```python
from build123d import *

# Parameters (mm, degrees)
ESBO_O1_R                      = 1.5
RESSALTO_EXTRUS_O1_DEPTH       = 6
ESBO_O6_W                      = 14
ESBO_O6_H                      = 22
RESSALTO_EXTRUS_O3_DEPTH       = 12
ESBO_O7_R                      = 5
CORTE_EXTRUS_O4_DEPTH          = 30.538450843
FILETE3_R                      = 5
RESSALTO_EXTRUS_O13_DEPTH      = 8
RESSALTO_EXTRUS_O13_DEPTH_BACK = 5
ESBO_O15_R                     = 2
ESBO_O17_R                     = 1
CORTE_EXTRUS_O6_DEPTH          = 8
ESBO_O21_W                     = 22.669500521
ESBO_O21_H                     = 31.157259519
CORTE_EXTRUS_O8_DEPTH          = 6
ESBO_O22_W                     = 5
ESBO_O22_H                     = 5
ESBO_O22_R                     = 1.5
RESSALTO_EXTRUS_O15_DEPTH      = 3
ESBO_O23_R                     = 2.5
RESSALTO_EXTRUS_O16_DEPTH      = 5
ESBO_O24_R                     = 0.75
CORTE_EXTRUS_O9_DEPTH          = 5
CHANFRO5_SIZE                  = 1
ESBO_O25_R                     = 1.5
CORTE_EXTRUS_O11_DEPTH         = 14


with BuildPart() as part:
    # Esboço1 → Ressalto-extrusão1 (new body)
    with BuildSketch(Plane.XY):
        Polygon((-11.637137788, -1.832768542), (5.362862212, -1.832768542), (5.362862212, 7.667231458), (10.362862212, 7.667231458), (10.362862212, 16.667231458), (5.362862212, 16.667231458), (5.362862212, 20.167231458), (-10.637137788, 20.167231458), (-10.637137788, 16.667231458), (-15.637137788, 16.667231458), (-15.637137788, 7.667231458), (-11.637137788, 7.667231458), align=None)
        with Locations((6.362862212, 11.867231458)):
            Circle(ESBO_O1_R, mode=Mode.SUBTRACT)
        with Locations((-11.637137788, 11.867231458)):
            Circle(ESBO_O1_R, mode=Mode.SUBTRACT)
    extrude(amount=RESSALTO_EXTRUS_O1_DEPTH)

    # Esboço6 → Ressalto-extrusão3 (add)
    with BuildSketch(Plane(origin=(0, 0, 0), x_dir=(-1, 0, 0), z_dir=(0, 0, -1))):
        with Locations((2.637137788, 9.167231458)):
            Rectangle(ESBO_O6_W, ESBO_O6_H)
    extrude(amount=RESSALTO_EXTRUS_O3_DEPTH)

    # Esboço7 → Corte-extrusão4 (cut, through all)
    with BuildSketch(Plane.XZ.offset(1.832768542)):
        with Locations(Location((-2.637137788, -5, 0), (0, 0, 270))):
            Circle(ESBO_O7_R)
    extrude(amount=-CORTE_EXTRUS_O4_DEPTH, mode=Mode.SUBTRACT)

    # Filete3
    filete3_edges = [part.edges().sort_by_distance(p)[0] for p in [
        (4.362862212, 9.167231458, -12),
        (-9.637137788, 9.167231458, -12),
    ]]
    fillet(filete3_edges, radius=FILETE3_R)

    # Esboço15 → Ressalto-extrusão13 (add, two sides: drawn at the far end of the back side and taken through both)
    with BuildSketch(Plane(origin=(0, 20.167231458, 0), x_dir=(1, 0, 0), z_dir=(0, 1, 0)).offset(-RESSALTO_EXTRUS_O13_DEPTH_BACK)):
        with Locations(Location((-8.650480796, 5, 0), (0, 0, 270))):
            Circle(ESBO_O15_R)
        with Locations(Location((3.376205221, 5, 0), (0, 0, 270))):
            Circle(ESBO_O15_R)
    extrude(amount=RESSALTO_EXTRUS_O13_DEPTH + RESSALTO_EXTRUS_O13_DEPTH_BACK)

    # Esboço17 → Corte-extrusão6 (cut)
    with BuildSketch(Plane(origin=(0, 28.167231458, 0), x_dir=(1, 0, 0), z_dir=(0, 1, 0))):
        with Locations(Location((-8.650480796, 5, 0), (0, 0, 270))):
            Circle(ESBO_O17_R)
        with Locations(Location((3.376205221, 5, 0), (0, 0, 270))):
            Circle(ESBO_O17_R)
    extrude(amount=-CORTE_EXTRUS_O6_DEPTH, mode=Mode.SUBTRACT)

    # Esboço21 → Corte-extrusão8 (cut)
    with BuildSketch(Plane(origin=(0, 0, -7.115225733), x_dir=(1, 0, 0), z_dir=(0, 0, -1))):
        with Locations((-2.778124877, -9.864448806)):
            Rectangle(ESBO_O21_W, ESBO_O21_H)
    extrude(amount=CORTE_EXTRUS_O8_DEPTH, mode=Mode.SUBTRACT)

    # Esboço22 → Ressalto-extrusão15 (add)
    # profile 1 of 2: a face of its own
    with BuildSketch(Plane(origin=(0, 0, -7.115225733), x_dir=(1, 0, 0), z_dir=(0, 0, -1))):
        with Locations((-12.135809914, -15.625880271)):
            Rectangle(ESBO_O22_W, ESBO_O22_H)
        with Locations(Location((-12.135809914, -15.625880271, 0), (0, 0, 180))):
            Circle(ESBO_O22_R, mode=Mode.SUBTRACT)
    # profile 2 of 2: a face of its own
    with BuildSketch(Plane(origin=(0, 0, -7.115225733), x_dir=(1, 0, 0), z_dir=(0, 0, -1))):
        with Locations((6.862862212, -15.625880271)):
            Rectangle(ESBO_O22_W, ESBO_O22_H)
        with Locations(Location((6.862862212, -15.625880271, 0), (0, 0, 180))):
            Circle(ESBO_O22_R, mode=Mode.SUBTRACT)
    extrude(amount=-RESSALTO_EXTRUS_O15_DEPTH)

    # Esboço23 → Ressalto-extrusão16 (add)
    with BuildSketch(Plane.XZ.offset(1.832768542)):
        with Locations(Location((-9.213137788, 2.7, 0), (0, 0, 165.836166317))):
            Circle(ESBO_O23_R)
    extrude(amount=RESSALTO_EXTRUS_O16_DEPTH)

    # Esboço24 → Corte-extrusão9 (cut)
    with BuildSketch(Plane.XZ.offset(6.832768542)):
        with Locations(Location((-9.213137788, 2.7, 0), (0, 0, 270))):
            Circle(ESBO_O24_R)
    extrude(amount=-CORTE_EXTRUS_O9_DEPTH, mode=Mode.SUBTRACT)

    # Chanfro5
    # the kernel refuses this chamfer: 1 mm, written as the material it takes off along each edge
    with BuildSketch(Plane(origin=(6.362862212, 11.867231458, 0), x_dir=(1, 0, 0), z_dir=(0, -1, 0))) as chanfro5_piece_1_section:
        Polygon((1.5 + CHANFRO5_SIZE, 0), (1.5, CHANFRO5_SIZE), (1.5, 0), align=None)
    chanfro5_piece_1 = revolve(axis=Axis((6.362862212, 11.867231458, 0), (0, 0, 1)), mode=Mode.PRIVATE)
    chanfro5_piece_1 = split(chanfro5_piece_1, bisect_by=Plane(origin=(4.362862212, 13.893105183, 0.134898453), z_dir=(1, 0, 0)), keep=Keep.TOP, mode=Mode.PRIVATE)
    add(chanfro5_piece_1, mode=Mode.SUBTRACT)
    with BuildSketch(Plane(origin=(-11.637137788, 11.867231458, 0), x_dir=(1, 0, 0), z_dir=(0, -1, 0))) as chanfro5_piece_2_section:
        Polygon((1.5 + CHANFRO5_SIZE, 0), (1.5, CHANFRO5_SIZE), (1.5, 0), align=None)
    chanfro5_piece_2 = revolve(axis=Axis((-11.637137788, 11.867231458, 0), (0, 0, 1)), mode=Mode.PRIVATE)
    chanfro5_piece_2 = split(chanfro5_piece_2, bisect_by=Plane(origin=(-9.637137788, 11.867231458, 0.487087965), z_dir=(-1, 0, 0)), keep=Keep.TOP, mode=Mode.PRIVATE)
    add(chanfro5_piece_2, mode=Mode.SUBTRACT)

    # Esboço25 → Corte-extrusão11 (cut)
    with BuildSketch(Plane.ZY.offset(9.637137788)):
        with Locations((-1.5, 16.167231458)):
            Circle(ESBO_O25_R)
    extrude(amount=-CORTE_EXTRUS_O11_DEPTH, mode=Mode.SUBTRACT)


solid = part.part
```
Verification items for the finished model (mm, model axes). A direction names the side the tool comes from. Give positions to 0.01 mm unless a question says otherwise; leave off trailing zeros. Loops run counter-clockwise (first coordinate to the right, second up) from the corner with the lowest first, then second, coordinate; pieces in that order, holes last.
1. Section check B-B, the plane y = 7. Enter the section's corners in (x, z).
2. Thickness scan on line 1 (X direction, y = 26.75, z = -5); line 2 (Y direction, x = 8.75, z = 3.25); line 3 (Z direction, x = 3.5, y = 24). Record the ranges inside material, lowest first.
3. Go/stop test with flat-tipped pins: pin 1 Ø0.9 at (x, z) = (-9.21, 2.7) entering from -Y; pin 2 Ø4 at (y, z) = (-3, 1.5) entering from -X; pin 3 Ø2.5 at (x, z) = (-12, 1.5) entering from +Y. Record where each tip stops, or that it passes through.
4. Section check A-A, the plane z = -1.5. Enter the section's corners in (x, y).
5. Set-up check for faces 1 (the flat face through (9.363, 16, -6)), 2 (the cylindrical face through (-8.58, -4.37, 2.3)), 3 (the flat face through (4.7, 15.167, -3.8)): record each of +Z, -Z, +X, -X, +Y, -Y from which the full face is reachable in a straight line by a thin tool's end or side.
6. Section check D-D, the plane z = 2.7. Enter the section's corners in (x, y).
7. Mould release check, pull along Y, two halves, no side actions. Record for faces 4 (the conical face through (-13.295, 11.94, 0.84)), 5 (the flat face through (3, 20.167, -5)), 6 (the flat face through (-9.9, 15.167, -3.8)): released by +Y, released by -Y, zero draft, split by the parting line, or undercut.
8. Section check C-C, the plane x = 3. Enter the section's corners in (y, z).
Geometry says:
1. outline: (-11.64, 0) - (-9.64, 0) - (-9.64, -7) arc R5 ccw to (-9.64, -7.12) - (-7.17, -7.12) arc R5 cw (long way) to (1.89, -7.12) - (4.36, -7.12) arc R5 ccw to (4.36, -7) - (4.36, 0) - (5.36, 0) - (5.36, 6) - (-11.64, 6) - close
2. line 1: x = -10.65 to -9.65, -7.65 to -6.65, 1.38 to 2.38, 4.38 to 5.38
2. line 2: y = 7.67 to 16.67
2. line 3: z = -7 to -5.99, -4.01 to -3
3. pin 1: stops at y = -1.83
3. pin 2: stops at x = -11.71
3. pin 3: stops at y = 16.67
4. outline: (-9.64, -1.83) - (-6.21, -1.83) - (-6.21, 14.67) - (-9.64, 14.67) - close; (-9.64, 17.67) - (-6.21, 17.67) - (-6.21, 20.17) - (-9.64, 20.17) - close; (0.93, -1.83) - (4.36, -1.83) - (4.36, 14.67) - (0.93, 14.67) - close; (0.93, 17.67) - (4.36, 17.67) - (4.36, 20.17) - (0.93, 20.17) - close
5. face 1: -Z, +X, +Y, -Y
5. face 2: -Y
5. face 3: +X, -Y
6. outline: (-15.64, 7.67) - (-11.64, 7.67) - (-11.64, -1.83) - (-11.71, -1.83) - (-11.71, -6.83) - (-9.96, -6.83) - (-9.96, -1.83) - (-8.46, -1.83) - (-8.46, -6.83) - (-6.71, -6.83) - (-6.71, -1.83) - (5.36, -1.83) - (5.36, 7.67) - (10.36, 7.67) - (10.36, 16.67) - (5.36, 16.67) - (5.36, 20.17) - (-10.64, 20.17) - (-10.64, 16.67) - (-15.64, 16.67) - close; hole circle Ø3 at (-11.64, 11.87); hole circle Ø3 at (6.36, 11.87)
7. face 4: undercut
7. face 5: released by +Y
7. face 6: released by -Y
8. outline: (-1.83, -7.12) - (20.17, -7.12) - (20.17, -6.96) - (28.17, -6.96) - (28.17, -5.93) - (20.17, -5.93) - (20.17, -4.07) - (28.17, -4.07) - (28.17, -3.04) - (20.17, -3.04) - (20.17, 6) - (-1.83, 6) - close; hole circle Ø3 at (16.17, -1.5)
